Autodesk Inventor part; units mm, degrees
ref_plane "YZ Plane" through (0, 0, 0) normal (1, 0, 0) x (0, 1, 0)
ref_plane "XZ Plane" through (0, 0, 0) normal (0, 1, 0) x (-1, 0, 0)
ref_plane "XY Plane" through (0, 0, 0) normal (0, 0, 1) x (1, 0, 0)
sketch "Sketch1" plane through (0, 0, 0) normal (0, 0, 1) x (1, 0, 0)
  line L0 (0, 0) -> (41.275, 0)
  line L1 (41.275, 0) -> (41.275, 41.275)
  line L2 (41.275, 41.275) -> (0, 41.275)
  line L3 (0, 41.275) -> (0, 0)
  circle A0 centre (20.6375, 20.6375) radius 22.225 construction
  line L4 (0, 0) -> (41.275, 41.275) construction
  line L5 (0, 41.275) -> (41.275, 0) construction
  circle A1 centre (4.9221, 36.3529) radius 1.5875
  circle A2 centre (4.9221, 4.9221) radius 1.5875
  circle A3 centre (36.3529, 36.3529) radius 1.5875
  circle A4 centre (36.3529, 4.9221) radius 1.5875
  dimension "d0" = 41.275
  dimension "d2" = 41.275
  dimension "d3" = 44.45
  dimension "d4" = 3.175
  dimension "d5" = 3.175
  dimension "d6" = 3.175
  dimension "d7" = 3.175
  dimension "d8" = 20.6375
  dimension "d9" = 20.6375
extrude "Extrusion1" add sketch "Sketch1" along normal blind 6.35
sketch "Sketch2" plane through (0, 41.275, 0) normal (0, 1, 0) x (1, 0, 0)
  line L0 (41.275, 0) -> (0, 0)
  line L1 (0, 0) -> (0, -6.35)
  line L2 (41.275, 0) -> (41.275, -6.35)
  circle A0 centre (10.16, -3.175) radius 1.5964
  circle A1 centre (31.115, -3.175) radius 1.5964
  dimension "d12" = 3.1928
  dimension "d14" = 3.1928
  dimension "d15" = 10.16
  dimension "d17" = 10.16
  dimension "d18" = 3.175
  dimension "d19" = 3.175
extrude "Extrusion2" cut sketch "Sketch2" against normal blind 6.35
sketch "Sketch3" plane through (0, 0, 6.35) normal (0, 0, 1) x (1, 0, 0)
  line L0 (7.9375, 7.9375) -> (33.3375, 7.9375)
  line L1 (33.3375, 7.9375) -> (33.3375, 33.3375)
  line L2 (33.3375, 33.3375) -> (7.9375, 33.3375)
  line L3 (7.9375, 33.3375) -> (7.9375, 7.9375)
extrude "Extrusion3" cut sketch "Sketch3" against normal blind 3.175
fillet "Fillet1" radius 7.9375 1 edges at (7.9375, 33.3375, 4.7625)
fillet "Fillet2" radius 7.9375 3 edges at (7.9375, 7.9375, 4.7625) (33.3375, 7.9375, 4.7625) (33.3375, 33.3375, 4.7625)
sketch "Sketch4" plane through (0, 0, 3.175) normal (0, 0, 1) x (1, 0, 0)
  circle A0 centre (20.6375, 20.6375) radius 3.175
  point P0 (0, 0)
  dimension "d33" = 6.35
extrude "Extrusion4" cut sketch "Sketch4" against normal blind 25.4
properties part number "motor_mount"
Geometry: final body of the model. Coordinates: model frame, mm. A direction names the side the tool comes from. Coordinates: 2 decimals unless noted, no trailing zeros. Write each loop counter-clockwise with the first axis right and the second up, starting at its lowest first coordinate (ties: lowest second). Pieces come first, ordered by that corner, then holes. Notation, with made-up numbers: M 3.5,38 L 20.5,38 A31 ccw 20.5,73 Z; hole C -11,-18.5 d5. An arc over 180 degrees is marked long. Answer as CSV lines item,"result". Start each with the question number.
Q1. Line query: line 1 (Y direction, x = 5, z = 1.75) (3 decimals); line 2 (Y direction, x = 20, z = 4.5) (1 decimal); line 3 (X direction, y = 36, z = 2.25) (3 decimals). Output: solid intervals per line, ascending. Write a range as from..to.
Q2. Cut plane D-D on x = 10.16. Return the cut outline in (y, z) (3 decimals), then the cut area to 3 significant figures.
Q3. Mould query, pull axis Z, two halves, no side actions, for faces 1 (the cylindrical face through (32.64, 38.14, 2.7)), 2 (the flat face through (20, 26, 0)), 3 (the flat face through (20, 0, 3)), 4 (the flat face through (10, 34.925, 3)). Classes: released by +Z, released by -Z, zero draft, split by the parting line, or undercut.
Q4. Reachability of faces 5 (the cylindrical face through (5.655, 6.33, 3.131)), 6 (the flat face through (33.338, 21, 5)), 7 (the flat face through (31, 34.925, 3)) from +Z, -Z, +X, -X, +Y, -Y: full face, straight path, thin tool, end or side. Return the list, or none.
Q5. Pin query (flat end, axial travel): P1, Ø7.5, axis at x = 15.5, y = 26.5, coming from the +Z side (3 decimals). Return the tip coordinate at first contact, or that it passes through.
Q6. Cut plane C-C on z = 2.5. Count the separate pieces of the cut face and the enclosed holes in it, then the cut area to 3 significant figures.
Findings below:
1,line 1,"y = 0..3.337, 6.508..34.767, 37.938..41.275"
1,line 2,"y = 0..7.9, 33.3..41.3"
1,line 3,"x = 0..3.374, 6.47..8.859, 11.461..29.814, 32.416..34.805, 37.901..41.275"
2,outline,"M 0,0 L 41.275,0 L 41.275,1.579 L 34.925,1.579 L 34.925,4.771 L 41.275,4.771 L 41.275,6.35 L 30.908,6.35 L 30.908,3.175 L 10.367,3.175 L 10.367,6.35 L 0,6.35 Z"
2,area,"177 mm2"
3,face 1,"undercut"
3,face 2,"released by -Z"
3,face 3,"zero draft"
3,face 4,"undercut"
4,face 5,"+Z, -Z"
4,face 6,"+Z"
4,face 7,"+Y"
5,P1,"stops at z = 3.175"
6,separate pieces,"1"
6,enclosed holes,"5"
6,area,"1,600 mm2"
